Can you work these out from the model? Positions are in its coordinate system, mm. A direction names the side the tool comes from. Round coordinates to 2 decimals unless told otherwise and drop trailing zeros. One line per question, with ' | ' between items.
```python
from build123d import *

# Parameters (mm, degrees)
FILLET1_R          = 2
SHELL2_OUTLINE_W   = 22.0070482
SHELL2_OUTLINE_H   = 22.0070482
SHELL2_DEPTH       = 6.5
SHELL2_DRAFT       = -16.3895403
SKETCH5_R          = 2.5
CUT_EXTRUDE1_DEPTH = 10


with BuildPart() as part:
    # Sketch3 → Loft1 section 0
    with BuildSketch(Plane(origin=(0, 8.5, 0), x_dir=(1, 0, 0), z_dir=(0, 1, 0))):
        with BuildLine():
            Line((15, -15), (-15, -15))
            Line((-15, -15), (-15, 15))
            Line((-15, 15), (15, 15))
            Line((15, 15), (15, -15))
        make_face()
    # Sketch2 → Loft1 section 1
    with BuildSketch(Plane(origin=(0, 0, 0), x_dir=(1, 0, 0), z_dir=(0, 1, 0))):
        with BuildLine():
            Line((12.5, -12.5), (-12.5, -12.5))
            Line((-12.5, -12.5), (-12.5, 12.5))
            Line((-12.5, 12.5), (12.5, 12.5))
            Line((12.5, 12.5), (12.5, -12.5))
        make_face()
    loft()

    # Fillet1
    fillet1_edges = [part.edges().sort_by_distance(p)[0] for p in [
        (13.75, 4.25, -13.75),
        (-13.75, 4.25, -13.75),
        (-13.75, 4.25, 13.75),
        (13.75, 4.25, 13.75),
    ]]
    fillet(fillet1_edges, radius=FILLET1_R)


with BuildPart() as shell2_tool:
    # Shell2: read off the stored shape, not the designer's step
    # Shell2 outline → Shell2 (with draft: the straight prism first)
    with BuildSketch(Plane(origin=(0, 2, 0), x_dir=(1, 0, 0), z_dir=(0, 1, 0))):
        Rectangle(SHELL2_OUTLINE_W, SHELL2_OUTLINE_H)
    extrude(amount=SHELL2_DEPTH)
    # Shell2: the draft: its side faces are tilted about the plane it starts from
    shell2_sides = [shell2_tool.faces().sort_by_distance(p)[0] for p in [
        (0, 5.25, -11.0035241),
        (-11.0035241, 5.25, 0),
        (0, 5.25, 11.0035241),
        (11.0035241, 5.25, 0),
    ]]
    draft(shell2_sides, Plane(origin=(0, 2, 0), x_dir=(1, 0, 0), z_dir=(0, 1, 0)), SHELL2_DRAFT)


with BuildPart() as part_1:
    add(part.part)

    # Shell2: cut by shell2_tool
    add(shell2_tool.part, mode=Mode.SUBTRACT)

    # Sketch5 → Cut-Extrude1 (cut)
    with BuildSketch(Plane.XZ):
        with Locations(Location((0, 0, 0), (0, 0, 270))):
            Circle(SKETCH5_R)
    extrude(amount=-CUT_EXTRUDE1_DEPTH, mode=Mode.SUBTRACT)


solid = part_1.part
```
(1) Will these pins go through, and if not, where does the flat tip stop? pin 1 Ø4 at (y, z) = (6, 6) entering from -X; pin 2 Ø3 at (y, z) = (2, 7.5) entering from -X; pin 3 Ø4 at (x, y) = (-0.5, 2) entering from -Z; pin 4 Ø4 at (x, z) = (0, 0) entering from -Y.
Final values:
pin 1: x = -14.85 | pin 2: x = -13.53 | pin 3: z = -13.68 | pin 4: through
(2) Thinking about a two-plate mould opening in Z: for faces 1 (the flat face through (11.946, 5.205, 0.181)), 2 (the flat face through (1, 8.5, -14)), which applies, released by +Z, released by -Z, zero draft, split by the parting line, or undercut?
Final values:
face 1: undercut | face 2: zero draft
(3) On a 3-axis mill with a long thin cutter (end or side, diameter ignored), from which of +Z, -Z, +X, -X, +Y, -Y can I reach the whole of each face in a straight line? I mean faces 3 (the cylindrical face through (-2.44, 0.99, 0.54)), 4 (the flat face through (-0.181, 5.205, 11.946)). Say none if no direction works.
Final values:
face 3: +Y, -Y | face 4: +Y
(4) Please list where these lines run through material, in increasing order: probe 1 along Y at (x, z) = (-7.5, -4); probe 2 along X at (y, z) = (0.4, 0); probe 3 along X at (y, z) = (6.25, -11). Write a range as [from, to].
Final values:
probe 1: [0, 2] | probe 2: [-12.62, -2.5], [2.5, 12.62] | probe 3: [-14.34, -12.25], [12.25, 14.34]
